Autodesk Inventor part; units mm, degrees
ref_plane "YZ Plane" through (0, 0, 0) normal (1, 0, 0) x (0, 1, 0)
ref_plane "XZ Plane" through (0, 0, 0) normal (0, 1, 0) x (-1, 0, 0)
ref_plane "XY Plane" through (0, 0, 0) normal (0, 0, 1) x (1, 0, 0)
sketch "Sketch1" plane through (0, 0, 0) normal (0, 0, 1) x (1, 0, 0)
  line L0 (0, 0) -> (4, 0)
  line L1 (4, 0) -> (4, 6)
  line L2 (4, 6) -> (0, 6)
  line L3 (0, 6) -> (0, 0)
extrude "Extrusion1" add sketch "Sketch1" along normal blind 8
sketch "Sketch2" plane through (0, 0, 8) normal (0, 0, 1) x (1, 0, 0)
  line L0 (0.5, 0.5) -> (3.5, 0.5)
  line L1 (3.5, 0.5) -> (3.5, 5.5)
  line L2 (3.5, 5.5) -> (0.5, 5.5)
  line L3 (0.5, 5.5) -> (0.5, 0.5)
  point P0 (0, 0)
extrude "Extrusion2" add sketch "Sketch2" along normal blind 8
fillet "Fillet1" radius 1.5 2 edges at (3.5, 5.5, 12) (0.5, 0.5, 12)
properties part number "button_press_fitting_new"
The listing builds one solid part. Answer for the finished solid, in the listing's coordinates (mm). A direction names the side the tool comes from. Round coordinates to 2 decimals unless told otherwise and drop trailing zeros. Write each loop counter-clockwise with the first axis right and the second up, starting at its lowest first coordinate (ties: lowest second). Pieces come first, ordered by that corner, then holes. Notation, with made-up numbers: (-30, 69.5) -> (-12, 69.5) arc R22 cw to (-12, 84.5) -> close; hole circle Ø11 at (53, 68). An arc over 180 degrees is marked (long way). Answer as a JSON object with one key per item and string values. Group by question number.
Q1. Section A-A (x = 3.2) is taken. Write down the section's boundary in (y, z), plus the area to 3 significant figures.
Q2. Straight lines are drawn through the part: line 1 along Y through (x, z) = (2, 14.75); line 2 along Z through (x, y) = (1.45, 0.5); line 3 along X through (y, z) = (3.1, 11). For each, find the intervals that lie inside material, in ascending order.
Q3. Section D-D (x = 0.3) is taken. Write down the section's boundary in (y, z).
Q4. Section C-C (z = 11.25) is taken. Write down the section's boundary in (x, y).
Q5. Each of these flat-tipped pins is pushed along its axis until it touches: pin 1 Ø0.8 at (x, z) = (1, 13.5) entering from +Y; pin 2 Ø3 at (y, z) = (4, 10.5) entering from -X; pin 3 Ø3 at (y, z) = (2, 14) entering from +X. Where does it stop, or does it pass through?
Q6. Which of the six approach directions +Z, -Z, +X, -X, +Y, -Y give full straight-line access (tool end or side, diameter ignored) to faces 1 (the face through (0.5, 4, 12)), 2 (the face through (3.07, 5.05, 12.06)), 3 (the face through (0.93, 0.95, 12.06)), 4 (the face through (1, 5.5, 12))?
Q7. Section B-B (y = 3.4) is taken. Write down the section's boundary in (x, z).
Check values:
{
 "1": {"outline": "(0, 0) -> (6, 0) -> (6, 8) -> (4.9, 8) -> (4.9, 16) -> (0.5, 16) -> (0.5, 8) -> (0, 8) -> close", "area": "83.2 mm^2"},
 "2": {"line 1": "0.5 to 5.5", "line 2": "0 to 8", "line 3": "0.5 to 3.5"},
 "3": {"outline": "(0, 0) -> (6, 0) -> (6, 8) -> (0, 8) -> close"},
 "4": {"outline": "(0.5, 2) arc R1.5 ccw to (2, 0.5) -> (3.5, 0.5) -> (3.5, 4) arc R1.5 ccw to (2, 5.5) -> (0.5, 5.5) -> close"},
 "5": {"pin 1": "y = 5.5", "pin 2": "x = 0.5", "pin 3": "x = 3.5"},
 "6": {"face 1": "+Z, -X, +Y, -Y", "face 2": "+Z, +X, +Y", "face 3": "+Z, -X, -Y", "face 4": "+Z, +X, -X, +Y"},
 "7": {"outline": "(0, 0) -> (4, 0) -> (4, 8) -> (3.5, 8) -> (3.5, 16) -> (0.5, 16) -> (0.5, 8) -> (0, 8) -> close"}
}
